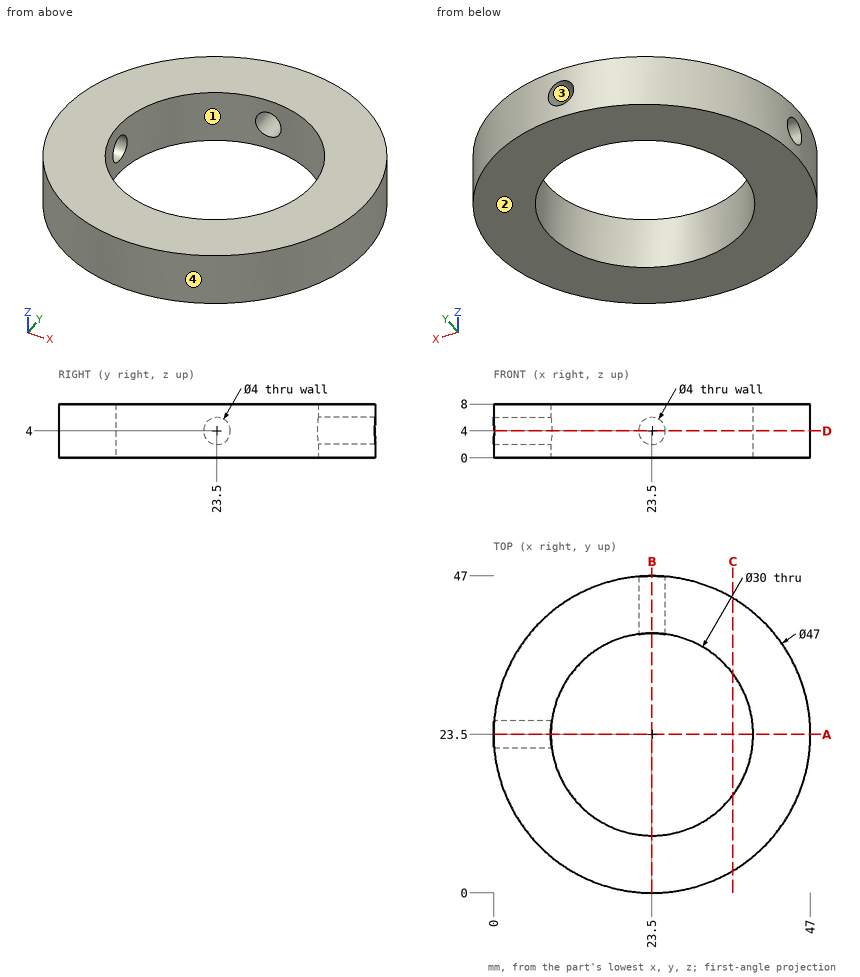
Geometry check sheet. Reference: drawing and pictorial views, mm from the part's lowest x, y, z. Round coordinates to 2 decimals unless told otherwise and drop trailing zeros. Write each loop counter-clockwise with the first axis right and the second up, starting at its lowest first coordinate (ties: lowest second). Pieces come first, ordered by that corner, then holes.
Item 1: Section check B-B (x = 23.5). Record the boundary of the cut face in (y, z).
Determined:
outline: (0, 0) - (8.5, 0) - (8.5, 8) - (0, 8) - close; (38.5, 0) - (47, 0) - (47, 2) - (38.5, 2) - close; (38.5, 6) - (47, 6) - (47, 8) - (38.5, 8) - close
Item 2: Material ranges on line 1 along Z through (x, y) = (23.5, 41); line 2 along Y through (x, z) = (23, 7.5); line 3 along X through (y, z) = (16, 4.5), recorded low to high.
Determined:
line 1: z = 0 to 2, 6 to 8
line 2: y = 0.01 to 8.51, 38.49 to 46.99
line 3: x = 1.23 to 10.51, 36.49 to 45.77
Item 3: Go/stop test with flat-tipped pins: pin 1 Ø12 at (x, y) = (11, 16.5) entering from +Z; pin 2 Ø3.5 at (x, z) = (23.5, 4) entering from +Y; pin 3 Ø1.5 at (y, z) = (32.5, 3) entering from +X; pin 4 Ø1.5 at (y, z) = (26, 1) entering from -X. Record where each tip stops, or that it passes through.
Determined:
pin 1: stops at z = 8
pin 2: stops at y = 8.6
pin 3: stops at x = 45.5
pin 4: stops at x = 0.07
Item 4: Mould release check, pull along X, two halves, no side actions. Record for the marked faces 1, 2, 3 and 4: +X half, -X half, draft (parallel to the pull), parting line (faces both ways), or undercut.
Determined:
face 1: undercut
face 2: draft
face 3: undercut
face 4: parting line
Item 5: Section check D-D (z = 4). Record the boundary of the cut face in (x, y).
Determined:
outline: (0.09, 21.5) arc R23.5 ccw (long way) to (25.5, 46.91) - (25.5, 38.37) arc R15 cw (long way) to (8.63, 21.5) - close; (0.09, 25.5) - (8.63, 25.5) arc R15 cw to (21.5, 38.37) - (21.5, 46.91) arc R23.5 ccw to start
Item 6: Section check C-C (x = 35.5). Record the boundary of the cut face in (y, z), plus the area to 3 significant figures.
Determined:
outline: (3.29, 0) - (14.5, 0) - (14.5, 8) - (3.29, 8) - close; (32.5, 0) - (43.71, 0) - (43.71, 8) - (32.5, 8) - close
area: 179 mm2
Item 7: Section check A-A (y = 23.5). Record the boundary of the cut face in (x, z).
Determined:
outline: (0, 0) - (8.5, 0) - (8.5, 2) - (0, 2) - close; (0, 6) - (8.5, 6) - (8.5, 8) - (0, 8) - close; (38.5, 0) - (47, 0) - (47, 8) - (38.5, 8) - close
